Geometry: final body of the model. Coordinates: model frame, mm. A direction names the side the tool comes from. Give positions to 0.01 mm unless a question says otherwise; leave off trailing zeros. Write each loop counter-clockwise with the first axis right and the second up, starting at its lowest first coordinate (ties: lowest second). Pieces come first, ordered by that corner, then holes. Notation, with made-up numbers: (87, -11.5) -> (95, -11.5) arc R16 ccw to (95, 7.5) -> close; hole circle Ø1 at (76.25, 45.25). An arc over 180 degrees is marked (long way). Use CSV: the item, a comma, the result in double quotes. Start each with the question number.
1) Material intervals for line 1 (Y direction, x = 4.25, z = -27); line 2 (X direction, y = -1, z = 1.5); line 3 (Z direction, x = -0.5, y = -10), sorted ascending. Write a range as [from, to].
2) Contact query for flat-ended pins moving along their axis: P1, Ø10, axis at x = -13.5, z = 2.5, coming from the +Y side; P2, Ø4, axis at x = -4.5, y = -9.5, coming from the +Z side; P3, Ø1, axis at x = 3.5, z = -16.5, coming from the -Y side. Output: stop coordinate, or through.
3) Set-up query: faces 4 (the face through (27, -18, -21.074)), 5 (the face through (9, 0, -9)), 6 (the face through (-23, 8, -21.074)). Return all of +Z, -Z, +X, -X, +Y, -Y with unobstructed straight access to the full face (end or side cutting, diameter ignored); none if empty.
4) Section C-C (x = -18.5). Output: boundary loops of the cut face in (y, z), plus the area to 3 significant figures.
5) Section B-B (y = -22.5). Output: boundary loops of the cut face in (x, z), plus the area to 3 significant figures.
6) Section A-A (z = 0). Output: boundary loops of the cut face in (x, y).
7) Section D-D (z = -34). Output: boundary loops of the cut face in (x, y), plus the area to 3 significant figures.
8) Draft query along X for faces 1 (the face through (-2.38, 2.96, -10.74)), 2 (the face through (25, -14, 0)), 3 (the face through (23, 8, -21.074)). Return one class per face: pulls with the +X half, pulls with the -X half, needs draft (parallel to the pull), parting line crosses it, or undercut.
```python
from build123d import *

# Parameters (mm, degrees)
F0_W     = 42
F0_H     = 42
F0_R     = 11
F1_DEPTH = 6
F0_W_2   = 4
F0_H_2   = 20
F2_DEPTH = 40
F3_DEPTH = 5
F4_DEPTH = 40
F6_R     = 1
F7_DEPTH = 25
F8_DEPTH = 12


with BuildPart() as f1:
    # F0 (on Front) → F1 (new body)
    with BuildSketch(Plane.XZ):
        Rectangle(F0_W, F0_H)
        with BuildLine():
            ThreePointArc((-15.5, 13.75), (-16.7374368671, 16.7374368671), (-13.75, 15.5))
            Line((-13.75, 15.5), (15.5, 15.5))
            Line((15.5, 15.5), (15.5, -13.75))
            ThreePointArc((15.5, -13.75), (16.7374368671, -14.2625631329), (17.25, -15.5))
            ThreePointArc((17.25, -15.5), (15.5, -17.25), (13.75, -15.5))
            Line((13.75, -15.5), (-13.75, -15.5))
            ThreePointArc((-13.75, -15.5), (-16.7374368671, -16.7374368671), (-15.5, -13.75))
            Line((-15.5, -13.75), (-15.5, 13.75))
        make_face(mode=Mode.SUBTRACT)
        with BuildLine():
            Line((15.5, 15.5), (-13.75, 15.5))
            ThreePointArc((-13.75, 15.5), (-14.2625631329, 14.2625631329), (-15.5, 13.75))
            Line((-15.5, 13.75), (-15.5, -13.75))
            ThreePointArc((-15.5, -13.75), (-14.2625631329, -14.2625631329), (-13.75, -15.5))
            Line((-13.75, -15.5), (13.75, -15.5))
            ThreePointArc((13.75, -15.5), (14.2625631329, -14.2625631329), (15.5, -13.75))
            Line((15.5, -13.75), (15.5, 15.5))
        make_face()
        Circle(F0_R, mode=Mode.SUBTRACT)
    extrude(amount=-F1_DEPTH)



with BuildPart() as f2:
    # F0 (on Front) → F2 (new body)
    with BuildSketch(Plane.XZ):
        with Locations((-23, -31.0743206739)):
            Rectangle(F0_W_2, F0_H_2)
        with Locations((0, -31.0743206739)):
            Rectangle(F0_W, F0_H_2)
        with Locations((23, -31.0743206739)):
            Rectangle(F0_W_2, F0_H_2)
        with Locations((27, -31.0743206739)):
            Rectangle(F0_W_2, F0_H_2)
    extrude(amount=F2_DEPTH)

    # F3 (add): a face of the model
    f3_faces = [f2.faces().sort_by_distance(p)[0] for p in [
        (2, 0, -31.0743206739),
    ]]
    extrude(f3_faces, amount=F3_DEPTH)


with BuildPart() as f1_1:
    add(f1.part)

    add(f2.part)  # F4 merges F2
    # F0 (on Front) → F4 (join)
    with BuildSketch(Plane.XZ):
        Polygon((-21, -21), (-21, 21), (-25, 21), (-25, -21.0743206739), (-21, -21.0743206739), align=None)
        with Locations((-23, -31.0743206739)):
            Rectangle(F0_W_2, F0_H_2)
        Polygon((25, 21), (21, 21), (21, -21), (21, -21.0743206739), (25, -21.0743206739), align=None)
        with Locations((23, -31.0743206739)):
            Rectangle(F0_W_2, F0_H_2)
    extrude(amount=F4_DEPTH)

    # F5: union 

    # F6 (on face) → F7 (cut)
    with BuildSketch(Plane.XY.offset(-21.0743206739)):
        with Locations((4.25, -22.5)):
            Circle(F6_R)
    extrude(amount=-F7_DEPTH, mode=Mode.SUBTRACT)

    # F8 (add): faces of the model
    f8_faces = [f1_1.faces().sort_by_distance(p)[0] for p in [
        (23, 0, -0.037160337),
        (-23, 0, -0.037160337),
    ]]
    extrude(f8_faces, amount=F8_DEPTH)


solid = f1_1.part
```
Answers follow:
1,line 1,"y = [-40, -23.5], [-21.5, 5]"
1,line 2,"x = [-25, -21], [21, 25]"
1,line 3,"z = [-41.07, -21.07]"
2,P1,"stops at y = 6"
2,P2,"stops at z = -21.07"
2,P3,"stops at y = 0"
3,face 4,"+Z, +X, +Y, -Y"
3,face 5,"+Z, -Y"
3,face 6,"-Z, +X, -X, +Y"
4,outline,"(-40, -41.07) -> (5, -41.07) -> (5, -21.07) -> (-40, -21.07) -> close; (0, -21) -> (6, -21) -> (6, 21) -> (0, 21) -> close"
4,area,"1,150 mm^2"
5,outline,"(-25, -41.07) -> (3.25, -41.07) -> (3.25, -21.07) -> (-21, -21.07) -> (-21, 21) -> (-25, 21) -> close; (5.25, -41.07) -> (29, -41.07) -> (29, -21.07) -> (25, -21.07) -> (25, 21) -> (21, 21) -> (21, -21.07) -> (5.25, -21.07) -> close"
5,area,"1,380 mm^2"
6,outline,"(-25, -40) -> (-21, -40) -> (-21, 0) -> (-11, 0) -> (-11, 6) -> (-21, 6) -> (-21, 12) -> (-25, 12) -> close; (11, 0) -> (21, 0) -> (21, -40) -> (25, -40) -> (25, 12) -> (21, 12) -> (21, 6) -> (11, 6) -> close"
7,outline,"(-25, -40) -> (29, -40) -> (29, 5) -> (-25, 5) -> close; hole circle Ø2 at (4.25, -22.5)"
7,area,"2,430 mm^2"
8,face 1,"undercut"
8,face 2,"pulls with the +X half"
8,face 3,"needs draft"
